Verification items for the finished model (mm, model axes). A direction names the side the tool comes from. Give positions to 0.01 mm unless a question says otherwise; leave off trailing zeros. Write each loop counter-clockwise with the first axis right and the second up, starting at its lowest first coordinate (ties: lowest second). Pieces come first, ordered by that corner, then holes. Notation, with made-up numbers: (-23, 80) - (15, 80) arc R29 cw to (15, 109) - close; hole circle Ø11 at (39.25, -10). An arc over 180 degrees is marked (long way). Put each result on its own line as item: value.
from build123d import *

# Parameters (mm, degrees)
SKETCH1_W           = 35
SKETCH1_H           = 35
SKETCH1_R           = 2.25
BOSS_EXTRUDE1_DEPTH = 5
FILLET1_R           = 4
SKETCH2_R           = 9.5
CUT_EXTRUDE1_DEPTH  = 3


with BuildPart() as part:
    # Sketch1 → Boss-Extrude1 (new body)
    with BuildSketch(Plane.XY):
        with Locations((-17.5, 239.7)):
            Rectangle(SKETCH1_W, SKETCH1_H)
        with Locations((-7, 250.2)):
            Circle(SKETCH1_R, mode=Mode.SUBTRACT)
        with Locations((-7, 229.2)):
            Circle(SKETCH1_R, mode=Mode.SUBTRACT)
        with Locations((-28, 229.2)):
            Circle(SKETCH1_R, mode=Mode.SUBTRACT)
        with Locations((-28, 250.2)):
            Circle(SKETCH1_R, mode=Mode.SUBTRACT)
    extrude(amount=BOSS_EXTRUDE1_DEPTH)

    # Fillet1
    fillet1_edges = [part.edges().sort_by_distance(p)[0] for p in [
        (0, 222.2, 2.5),
        (-35, 222.2, 2.5),
        (-35, 257.2, 2.5),
        (0, 257.2, 2.5),
    ]]
    fillet(fillet1_edges, radius=FILLET1_R)

    # Sketch2 → Cut-Extrude1 (cut)
    with BuildSketch(Plane(origin=(0, 0, 0), x_dir=(-1, 0, 0), z_dir=(0, 0, -1))):
        with Locations((17.5, 239.7)):
            Circle(SKETCH2_R)
    extrude(amount=-CUT_EXTRUDE1_DEPTH, mode=Mode.SUBTRACT)


solid = part.part
Q1. Scan lines: line 1 along Y through (x, z) = (-7, 4.55); line 2 along X through (y, z) = (229.2, 1.7); line 3 along Y through (x, z) = (-6, 2). Record each from-to range of solid material in increasing order.
Answers follow:
line 1: y = 222.2 to 226.95, 231.45 to 247.95, 252.45 to 257.2
line 2: x = -35 to -30.25, -25.75 to -9.25, -4.75 to 0
line 3: y = 222.2 to 227.18, 231.22 to 248.18, 252.22 to 257.2
Q2. Section check D-D, the plane x = -28. Record the cut outline in (y, z), plus the area to 3 significant figures.
Answers follow:
outline: (222.2, 0) - (226.95, 0) - (226.95, 5) - (222.2, 5) - close; (231.45, 0) - (247.95, 0) - (247.95, 5) - (231.45, 5) - close; (252.45, 0) - (257.2, 0) - (257.2, 5) - (252.45, 5) - close
area: 130 mm2
Q3. Release check for a two-part mould opening along Y. For faces 1 (the face through (-7.488, 227.004, 2.465)), 2 (the face through (-26, 232, 0)), 3 (the face through (-33.859, 223.403, 2.535)) record: released by +Y, released by -Y, zero draft, split by the parting line, or undercut.
Answers follow:
face 1: undercut
face 2: zero draft
face 3: released by -Y
Q4. Go/stop test with a flat-tipped pin: pin 1 Ø5 at (x, y) = (-7, 229.2) entering from +Z. Record where the tip stops, or that it passes through.
Answers follow:
pin 1: stops at z = 5
Q5. Section check A-A, the plane y = 250.2. Record the cut outline in (x, z).
Answers follow:
outline: (-35, 0) - (-30.25, 0) - (-30.25, 5) - (-35, 5) - close; (-25.75, 0) - (-9.25, 0) - (-9.25, 5) - (-25.75, 5) - close; (-4.75, 0) - (0, 0) - (0, 5) - (-4.75, 5) - close
Q6. Section check B-B, the plane z = 0.5. Record the cut outline in (x, y).
Answers follow:
outline: (-35, 226.2) arc R4 ccw to (-31, 222.2) - (-4, 222.2) arc R4 ccw to (0, 226.2) - (0, 253.2) arc R4 ccw to (-4, 257.2) - (-31, 257.2) arc R4 ccw to (-35, 253.2) - close; hole circle Ø4.5 at (-28, 229.2); hole circle Ø4.5 at (-28, 250.2); hole circle Ø19 at (-17.5, 239.7); hole circle Ø4.5 at (-7, 229.2); hole circle Ø4.5 at (-7, 250.2)
Q7. Set-up check for faces 4 (the face through (-17, 240, 3)), 5 (the face through (-1.203, 256.059, 2.535)): record each of +Z, -Z, +X, -X, +Y, -Y from which the full face is reachable in a straight line by a thin tool's end or side.
Answers follow:
face 4: -Z
face 5: +Z, -Z, +X, +Y
Q8. Section check C-C, the plane x = -17.5. Record the cut outline in (y, z).
Answers follow:
outline: (222.2, 0) - (230.2, 0) - (230.2, 3) - (249.2, 3) - (249.2, 0) - (257.2, 0) - (257.2, 5) - (222.2, 5) - close
